Design review of the part built by this model. Coordinates are the model's own, in mm. Face numbers are marked on the shaded views. Coordinates: 2 decimals unless noted, no trailing zeros. Write each loop counter-clockwise with the first axis right and the second up, starting at its lowest first coordinate (ties: lowest second). Pieces come first, ordered by that corner, then holes.
Q1. For probe 1 along Z at (x, y) = (-84, 40.5); probe 2 along Z at (x, y) = (140.5, -6), list the stretches that pass through material, from the lowest coordinate up.
Q2. Take a section at A-A (y = -8). Give the boundary of the cut face in (x, z).
Q3. Insertion check: pin 1 (8 mm diameter, centred on x = -147.72, y = 31.75, fed in from -Z). The pin has a flat end and moves straight along its axis. Give the tip position at first contact, or say it passes through.
Q4. Mouldability with a two-part tool opening along X and no side actions: class the marked faces 1, 2, 3 and 4 as pulls with the +X half, pulls with the -X half, needs draft (parallel to the pull), parting line crosses it, or undercut.
Q5. Take a section at C-C (z = 117). Give the boundary of the cut face in (x, y).
Q6. Take a section at B-B (x = -9). Give the boundary of the cut face in (y, z).
Q7. Take a section at D-D (x = -140). Give the boundary of the cut face in (y, z).
```python
from build123d import *

# Parameters (mm, degrees)
SKETCH1_W                                  = 381
SKETCH1_H                                  = 381
SKETCH1_W_2                                = 355.6
SKETCH1_H_2                                = 355.6
BOSS_EXTRUDE2_DEPTH                        = 50.8
SKETCH2_R                                  = 2.54
CUT_EXTRUDE3_DEPTH                         = 418.750858766
MIRROR1_AT_THE_SECOND_PLANE_COPY_1_SKETC_R = 2.54
MIRROR1_AT_THE_SECOND_PLANE_COPY_1_DEPTH   = 418.750858766
SKETCH3_W                                  = 381
SKETCH3_H                                  = 381
BOSS_EXTRUDE3_DEPTH                        = 12.7
CUT_EXTRUDE4_DEPTH                         = 275.155320941


with BuildPart() as part:
    # Sketch1 → Boss-Extrude2 (new body)
    with BuildSketch(Plane(origin=(0, 0, 0), x_dir=(1, 0, 0), z_dir=(0, 1, 0))):
        Rectangle(SKETCH1_W, SKETCH1_H)
        Rectangle(SKETCH1_W_2, SKETCH1_H_2, mode=Mode.SUBTRACT)
    extrude(amount=BOSS_EXTRUDE2_DEPTH)

    # Sketch2 → Cut-Extrude3 (cut, through all)
    with BuildSketch(Plane.XY.offset(-177.8)):
        with Locations((-147.717881469, 31.75)):
            Circle(SKETCH2_R)
    cut_extrude3 = extrude(amount=-CUT_EXTRUDE3_DEPTH, mode=Mode.SUBTRACT)

    # Mirror1: Cut-Extrude3 across plane
    add(cut_extrude3.mirror(Plane.XY), mode=Mode.SUBTRACT)

    # Mirror1 at the second plane: Cut-Extrude3 across plane
    add(cut_extrude3.mirror(Plane(origin=(0, 0, 0), x_dir=(0, 0, 1), z_dir=(1, 0, 0))), mode=Mode.SUBTRACT)

    # Mirror1 at the second plane copy 1 sketc → Mirror1 at the second plane copy 1 (cut, through all)
    with BuildSketch(Plane(origin=(0, 0, 177.8), x_dir=(-1, 0, 0), z_dir=(0, 0, -1))):
        with Locations((-147.717881469, 31.75)):
            Circle(MIRROR1_AT_THE_SECOND_PLANE_COPY_1_SKETC_R)
    extrude(amount=-MIRROR1_AT_THE_SECOND_PLANE_COPY_1_DEPTH, mode=Mode.SUBTRACT)

    # Sketch3 → Boss-Extrude3 (add)
    with BuildSketch(Plane.XZ):
        Rectangle(SKETCH3_W, SKETCH3_H)
    extrude(amount=BOSS_EXTRUDE3_DEPTH)

    # Sketch4 → Cut-Extrude4 (cut, through all)
    with BuildSketch(Plane(origin=(0, 0, 0), x_dir=(1, 0, 0), z_dir=(0, 1, 0))):
        Polygon((-152.4, 165.1), (0, 25.4), (152.4, 165.1), align=None)
        Polygon((165.1, 152.4), (165.1, -152.4), (25.4, 0), align=None)
        Polygon((152.4, -165.1), (-152.4, -165.1), (0, -25.4), align=None)
        Polygon((-165.1, -152.4), (-165.1, 152.4), (-25.4, 0), align=None)
    extrude(amount=-CUT_EXTRUDE4_DEPTH, mode=Mode.SUBTRACT)


solid = part.part
```
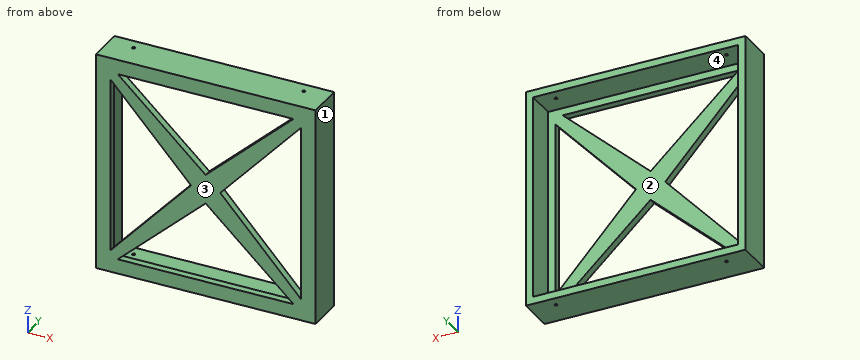
Response:
1. probe 1: z = -190.5 to -177.8, 177.8 to 190.5
1. probe 2: z = -190.5 to -165.1, -154.19 to -125.56, 125.56 to 154.19, 165.1 to 190.5
2. outline: (-190.5, -190.5) - (190.5, -190.5) - (190.5, 190.5) - (-190.5, 190.5) - close; hole (-165.1, -152.4) - (-25.4, 0) - (-165.1, 152.4) - close; hole (-152.4, -165.1) - (152.4, -165.1) - (0, -25.4) - close; hole (-152.4, 165.1) - (0, 25.4) - (152.4, 165.1) - close; hole (25.4, 0) - (165.1, -152.4) - (165.1, 152.4) - close
3. pin 1: stops at z = -190.5
4. face 1: pulls with the +X half
4. face 2: undercut
4. face 3: needs draft
4. face 4: undercut
5. outline: (-190.5, -12.7) - (-165.1, -12.7) - (-165.1, 0) - (-177.8, 0) - (-177.8, 50.8) - (-190.5, 50.8) - close; (-132.65, -12.7) - (-99.93, -12.7) - (-99.93, 0) - (-132.65, 0) - close; (99.93, -12.7) - (132.65, -12.7) - (132.65, 0) - (99.93, 0) - close; (165.1, -12.7) - (190.5, -12.7) - (190.5, 50.8) - (177.8, 50.8) - (177.8, 0) - (165.1, 0) - close
6. outline: (-12.7, -190.5) - (50.8, -190.5) - (50.8, -177.8) - (0, -177.8) - (0, -165.1) - (-12.7, -165.1) - close; (-12.7, -33.65) - (0, -33.65) - (0, 33.65) - (-12.7, 33.65) - close; (-12.7, 165.1) - (0, 165.1) - (0, 177.8) - (50.8, 177.8) - (50.8, 190.5) - (-12.7, 190.5) - close
7. outline: (-12.7, -190.5) - (50.8, -190.5) - (50.8, -177.8) - (0, -177.8) - (0, -165.1) - (-12.7, -165.1) - close; (-12.7, -153.73) - (0, -153.73) - (0, -125.02) - (-12.7, -125.02) - close; (-12.7, 125.02) - (0, 125.02) - (0, 153.73) - (-12.7, 153.73) - close; (-12.7, 165.1) - (0, 165.1) - (0, 177.8) - (50.8, 177.8) - (50.8, 190.5) - (-12.7, 190.5) - close
